Can you work these out from the drawing? Everything is in mm from the part's minimum corner. Give positions to 0.01 mm unless a question says otherwise; leave off trailing zeros. Loops run counter-clockwise (first coordinate to the right, second up) from the corner with the lowest first, then second, coordinate; pieces in that order, holes last. Notation, with made-up numbers: (27, 79) - (35, 79) arc R24 cw to (35, 110) - close; hole circle Ø2 at (64.5, 6.5). An arc over 180 degrees is marked (long way). Answer in a Markdown table with one row per item.
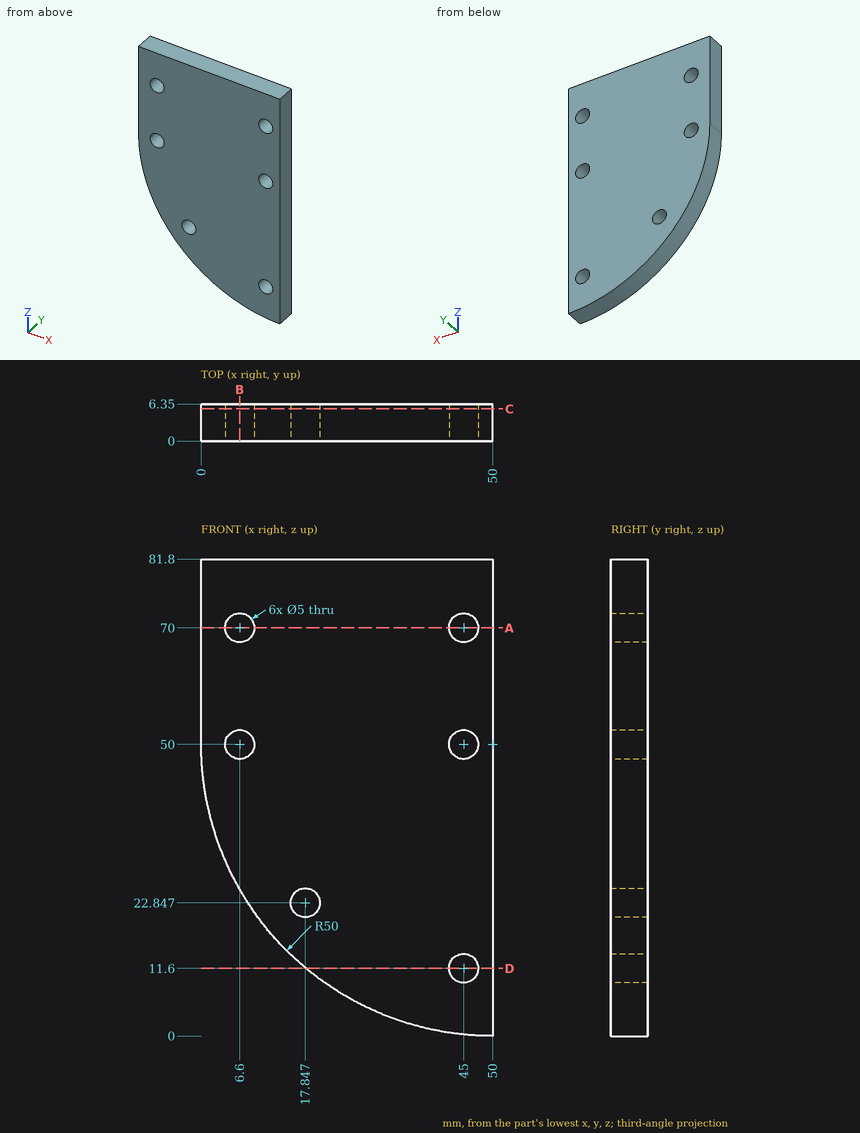
Q1. If I drill on line 1 (X direction, y = 4.5, z = 70); line 2 (Z direction, x = 5, y = 3.75) (1 decimal); line 3 (Z direction, x = 7.5, y = 3), over which ranges is the centre line in solid material (lowest first)? Write a range as [from, to].
Checked values:
| item | result |
|---|---|
| line 1 | x = [0, 4.1], [9.1, 42.5], [47.5, 50] |
| line 2 | z = [28.2, 48.1], [51.9, 68.1], [71.9, 81.8] |
| line 3 | z = [23.66, 47.67], [52.33, 67.67], [72.33, 81.8] |
Q2. Imagine slicing it at C-C, the plane y = 5.5. Write out the boundary of the cut face in (x, z), and give its area (3 significant figures).
Checked values:
| item | result |
|---|---|
| outline | (0, 50) arc R50 ccw to (50, 0) - (50, 81.8) - (0, 81.8) - close; hole circle Ø5 at (6.6, 50); hole circle Ø5 at (6.6, 70); hole circle Ø5 at (17.85, 22.85); hole circle Ø5 at (45, 11.6); hole circle Ø5 at (45, 50); hole circle Ø5 at (45, 70) |
| area | 3,440 mm² |
Q3. Imagine slicing it at A-A, the plane z = 70. Write out the boundary of the cut face in (x, y), and give its area (3 significant figures).
Checked values:
| item | result |
|---|---|
| outline | (0, 0) - (4.1, 0) - (4.1, 6.35) - (0, 6.35) - close; (9.1, 0) - (42.5, 0) - (42.5, 6.35) - (9.1, 6.35) - close; (47.5, 0) - (50, 0) - (50, 6.35) - (47.5, 6.35) - close |
| area | 254 mm² |
Q4. Imagine slicing it at B-B, the plane x = 6.6. Write out the boundary of the cut face in (y, z), and give its area (3 significant figures).
Checked values:
| item | result |
|---|---|
| outline | (0, 25.17) - (6.35, 25.17) - (6.35, 47.5) - (0, 47.5) - close; (0, 52.5) - (6.35, 52.5) - (6.35, 67.5) - (0, 67.5) - close; (0, 72.5) - (6.35, 72.5) - (6.35, 81.8) - (0, 81.8) - close |
| area | 296 mm² |
Q5. Imagine slicing it at D-D, the plane z = 11.6. Write out the boundary of the cut face in (x, y), and give its area (3 significant figures).
Checked values:
| item | result |
|---|---|
| outline | (17.98, 0) - (42.5, 0) - (42.5, 6.35) - (17.98, 6.35) - close; (47.5, 0) - (50, 0) - (50, 6.35) - (47.5, 6.35) - close |
| area | 172 mm² |
